The model under review builds one solid part; all positions refer to its coordinate system, in mm. Face numbers are marked on the shaded views. A direction names the side the tool comes from. Coordinates: 2 decimals unless noted, no trailing zeros. Order: outer loops, then holes, each group sorted by start corner. A loop starts at its lowest first (then second) coordinate and runs counter-clockwise, first axis right, second up. Notation, with made-up numbers: (51.25, 46) - (90.25, 46) arc R24 cw to (90.25, 76) - close; hole circle Ø1 at (65.25, 16.25). An arc over 180 degrees is marked (long way). Answer in a Markdown table with one row per item.
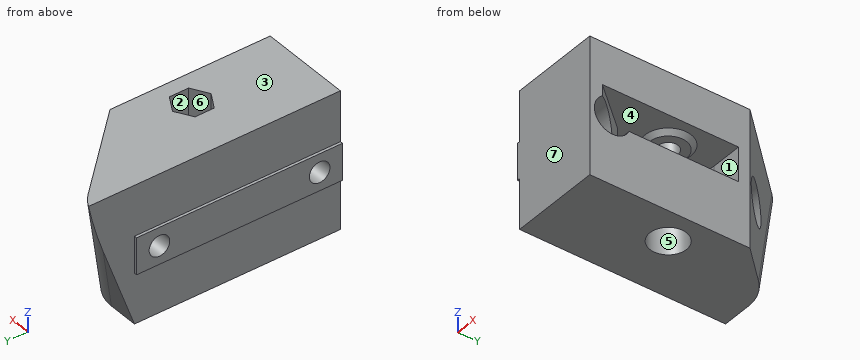
```python
from build123d import *

# Parameters (mm, degrees)
BOSS_EXTRUDE1_DEPTH = 22.5
CUT_EXTRUDE1_DEPTH  = 3.75
SKETCH3_R           = 2.15
CUT_EXTRUDE2_DEPTH  = 43.5
CUT_EXTRUDE3_DEPTH  = 7
SKETCH5_R           = 4
CUT_EXTRUDE4_DEPTH  = 8
CHAMFER4_START      = -3.75
CHAMFER4_DEPTH      = 7.5
SKETCH7_R           = 2.25
CUT_EXTRUDE5_DEPTH  = 35.922915113
CUT_EXTRUDE6_START  = -7
SKETCH8_R           = 4
CUT_EXTRUDE6_DEPTH  = 28.922915113
BOSS_EXTRUDE2_DEPTH = 20
CUT_EXTRUDE7_DEPTH  = 50.161333531
FILLET1_R           = 8
BOSS_EXTRUDE3_START = 1
SKETCH11_R          = 5
SKETCH11_R_2        = 2.15
BOSS_EXTRUDE3_DEPTH = 1
CHAMFER5_SIZE       = 1


with BuildPart() as part:
    # Sketch1 → Boss-Extrude1 (new, symmetric)
    with BuildSketch(Plane(origin=(0, 0, 0), x_dir=(1, 0, 0), z_dir=(0, 1, 0))):
        Polygon((0, -2), (0, -13), (20, -13), (20, 17), (0, 17), (0, 6), (-0.6, 6), (-0.6, -2), align=None)
    extrude(amount=BOSS_EXTRUDE1_DEPTH, both=True)

    # Sketch2 → Cut-Extrude1 (cut, symmetric)
    with BuildSketch(Plane.XY):
        with BuildLine():
            Line((13, 10), (20, 10))
            ThreePointArc((20, 10), (30, 0), (20, -10))
            Line((20, -10), (13, -10))
            ThreePointArc((13, -10), (3, 0), (13, 10))
        make_face()
    extrude(amount=CUT_EXTRUDE1_DEPTH, both=True, mode=Mode.SUBTRACT)

    # Sketch3 → Cut-Extrude2 (cut, through all)
    with BuildSketch(Plane(origin=(0, 0, -17), x_dir=(-1, 0, 0), z_dir=(0, 0, -1))):
        with Locations((-13, 0)):
            Circle(SKETCH3_R)
    extrude(amount=-CUT_EXTRUDE2_DEPTH, mode=Mode.SUBTRACT)

    # Sketch4 → Cut-Extrude3 (cut)
    with BuildSketch(Plane.XY.offset(13)):
        Polygon((13, -4.214656965), (16.65, -2.107328483), (16.65, 2.107328483), (13, 4.214656965), (9.35, 2.107328483), (9.35, -2.107328483), align=None)
    extrude(amount=-CUT_EXTRUDE3_DEPTH, mode=Mode.SUBTRACT)

    # Sketch5 → Cut-Extrude4 (cut)
    with BuildSketch(Plane(origin=(0, 0, -17), x_dir=(-1, 0, 0), z_dir=(0, 0, -1))):
        with Locations((-13, 0)):
            Circle(SKETCH5_R)
    extrude(amount=-CUT_EXTRUDE4_DEPTH, mode=Mode.SUBTRACT)

    # Chamfer4: read off the stored shape, not the designer's step
    # Chamfer4 outline → Chamfer4 (cut)
    with BuildSketch(Plane.XY.offset(CHAMFER4_START)):
        with BuildLine():
            ThreePointArc((13, -10), (12.247869581, -9.971674876), (11.5, -9.886859967))
            Line((11.5, -9.886859967), (20, -19.773719933))
            Line((20, -19.773719933), (20, -10))
            Line((20, -10), (13, -10))
        make_face()
    extrude(amount=CHAMFER4_DEPTH, mode=Mode.SUBTRACT)

    # Sketch7 → Cut-Extrude5 (cut, through all)
    with BuildSketch(Plane.ZY.offset(0.6)):
        with Locations((-2, 17.5)):
            Circle(SKETCH7_R)
        with Locations((-2, -17.5)):
            Circle(SKETCH7_R)
    extrude(amount=-CUT_EXTRUDE5_DEPTH, mode=Mode.SUBTRACT)

    # Sketch8 → Cut-Extrude6 (cut, through all)
    with BuildSketch(Plane.ZY.offset(0.6).offset(CUT_EXTRUDE6_START)):
        with Locations((-2, 17.5)):
            Circle(SKETCH8_R)
        with Locations((-2, -17.5)):
            Circle(SKETCH8_R)
    extrude(amount=-CUT_EXTRUDE6_DEPTH, mode=Mode.SUBTRACT)

    # Sketch9 → Boss-Extrude2 (add)
    with BuildSketch(Plane(origin=(20, 0, 0), x_dir=(0, 0, -1), z_dir=(1, 0, 0))):
        Polygon((17, 22.5), (-13, 22.5), (-13, 33.419107028), align=None)
    extrude(amount=-BOSS_EXTRUDE2_DEPTH)

    # Sketch10 → Cut-Extrude7 (cut, through all)
    with BuildSketch(Plane(origin=(0, 0, -17), x_dir=(-1, 0, 0), z_dir=(0, 0, -1))):
        Polygon((-20, 12.5), (-20, 33.419107028), (0, 33.419107028), align=None)
    extrude(amount=-CUT_EXTRUDE7_DEPTH, mode=Mode.SUBTRACT)

    # Fillet1
    fillet1_edges = [part.edges().sort_by_distance(p)[0] for p in [
        (5.219681229, 27.959553514, -2),
    ]]
    fillet(fillet1_edges, radius=FILLET1_R)

    # Sketch11 → Boss-Extrude3 (add)
    with BuildSketch(Plane(origin=(0, 0, 3.75), x_dir=(-1, 0, 0), z_dir=(0, 0, -1)).offset(BOSS_EXTRUDE3_START)):
        with Locations(Location((-13, 0, 0), (0, 0, 180))):
            Circle(SKETCH11_R)
        with Locations((-13, 0)):
            Circle(SKETCH11_R_2, mode=Mode.SUBTRACT)
    boss_extrude3 = extrude(amount=-BOSS_EXTRUDE3_DEPTH)

    # Mirror1: Boss-Extrude3 across plane
    add(boss_extrude3.mirror(Plane(origin=(0, 0, 0), x_dir=(1, 0, 0), z_dir=(0, 0, -1))))

    # Chamfer5
    chamfer5_edges = [part.edges().sort_by_distance(p)[0] for p in [
        (8, 0, 2.75),
        (8, 0, -2.75),
    ]]
    chamfer(chamfer5_edges, length=CHAMFER5_SIZE - 0.0001)  # a hair under: the kernel refuses the full size


solid = part.part
```
Item 1: Tool access review of the marked faces 4, 5, 6 and 7: name each direction out of +Z, -Z, +X, -X, +Y, -Y from which nothing blocks a thin tool from reaching the whole face with its end or side.
Check values:
| item | result |
|---|---|
| face 4 | none |
| face 5 | -Z |
| face 6 | +Z |
| face 7 | +Z, -Z, +X, -X, -Y |
Item 2: Mouldability with a two-part tool opening along Z and no side actions: class the marked faces 1, 2 and 3 as +Z half, -Z half, draft (parallel to the pull), parting line (faces both ways), or undercut.
Check values:
| item | result |
|---|---|
| face 1 | undercut |
| face 2 | draft |
| face 3 | +Z half |
Item 3: Clearance check with flat-ended pins moving along their axes: pin 1 Ø6.5 at (x, y) = (13, 0) entering from -Z; pin 2 Ø3 at (x, z) = (6.5, 6) entering from +Y; pin 3 Ø1.5 at (x, z) = (9.5, 4.5) entering from +Y; pin 4 Ø4 at (y, z) = (17.5, -2) entering from +X. State where each tip first meets the part, or that it passes through.
Check values:
| item | result |
|---|---|
| pin 1 | z = -9 |
| pin 2 | y = 28.18 |
| pin 3 | y = 24.27 |
| pin 4 | through |
Item 4: We need section C-C, the plane z = -2. State how many separate pieces and enclosed holes the cut face has, then the cut area to 3 significant figures.
Check values:
| item | result |
|---|---|
| separate pieces | 3 |
| enclosed holes | 0 |
| area | 356 mm^2 |
Item 5: To check wall thickness, follow line 1 (Z direction, x = 5.75, y = 6.5); line 2 (Y direction, x = 10.25, z = -2); line 3 (Z direction, x = 14.5, y = 17.5). State the ranges of each line that lie inside material, in increasing order. Write a range as from..to.
Check values:
| item | result |
|---|---|
| line 1 | -17..-3.75, 3.75..13 |
| line 2 | -22.5..-21.5, -13.5..-9.61, 9.61..13.5, 21.5..22.7 |
| line 3 | -17..-6, 2..13 |
Item 6: We need section B-B, the plane y = 11. Write out the cut boundary in (x, z), then the cut area to 3 significant figures.
Check values:
| item | result |
|---|---|
| outline | (-0.6, -6) - (0, -6) - (0, -17) - (20, -17) - (20, 13) - (0, 13) - (0, 2) - (-0.6, 2) - close |
| area | 605 mm^2 |
Item 7: We need section A-A, the plane y = -17.5. Write out the cut boundary in (x, z), then the cut area to 3 significant figures.
Check values:
| item | result |
|---|---|
| outline | (-0.6, -6) - (0, -6) - (0, -17) - (20, -17) - (20, -6) - (6.4, -6) - (6.4, -4.25) - (-0.6, -4.25) - close; (-0.6, 0.25) - (6.4, 0.25) - (6.4, 2) - (18.05, 2) - (18.05, 3.75) - (20, 3.75) - (20, 13) - (0, 13) - (0, 2) - (-0.6, 2) - close |
| area | 461 mm^2 |
